Design review of the part built by this model. Coordinates are the model's own, in mm. Face numbers are marked on the shaded views. A direction names the side the tool comes from. Coordinates: 2 decimals unless noted, no trailing zeros. Write each loop counter-clockwise with the first axis right and the second up, starting at its lowest first coordinate (ties: lowest second). Pieces come first, ordered by that corner, then holes.
Autodesk Inventor part; units mm, degrees
ref_plane "YZ Plane" through (0, 0, 0) normal (1, 0, 0) x (0, 1, 0)
ref_plane "XZ Plane" through (0, 0, 0) normal (0, 1, 0) x (-1, 0, 0)
ref_plane "XY Plane" through (0, 0, 0) normal (0, 0, 1) x (1, 0, 0)
sketch "Sketch1" plane through (0, 0, 0) normal (0, 1, 0) x (-1, 0, 0)
  line L0 (20, -4.85) -> (-20, -4.85) construction
  line L1 (-20, -4.85) -> (-20, 4.85) construction
  line L2 (-20, 4.85) -> (20, 4.85) construction
  line L3 (20, 4.85) -> (20, -4.85) construction
  line L4 (0, -4.85) -> (0, 4.85) construction
  line L5 (20, 0) -> (-20, 0) construction
  circle A0 centre (13.5, 0) radius 2.25
  circle A1 centre (-13.5, 0) radius 2.25
  line L6 (67, -18) -> (25, -18) construction
  line L7 (25, -18) -> (25, 18) construction
  line L8 (25, 18) -> (67, 18) construction
  line L9 (67, 18) -> (67, -18) construction
  line L10 (46, -18) -> (46, 18) construction
  line L11 (67, 0) -> (25, 0) construction
  circle A2 centre (61.25, -13) radius 2.75
  circle A3 centre (30.75, -13) radius 2.75
  circle A4 centre (61.25, 13) radius 2.75
  circle A5 centre (30.75, 13) radius 2.75
  line L12 (-67, -18) -> (-25, -18) construction
  line L13 (-25, -18) -> (-25, 18) construction
  line L14 (-25, 18) -> (-67, 18) construction
  line L15 (-67, 18) -> (-67, -18) construction
  line L16 (-46, -18) -> (-46, 18) construction
  line L17 (-67, 0) -> (-25, 0) construction
  circle A6 centre (-61.25, -13) radius 2.75
  circle A7 centre (-30.75, -13) radius 2.75
  circle A8 centre (-61.25, 13) radius 2.75
  circle A9 centre (-30.75, 13) radius 2.75
  line L18 (82, -65) -> (-82, -65)
  line L19 (-82, -65) -> (-82, 65)
  line L20 (-82, 65) -> (82, 65)
  line L21 (82, 65) -> (82, -65)
  point P0 (0, 0)
  point P1 (0, 0)
  dimension "d0" = 40
  dimension "d1" = 9.7
  dimension "d2" = 4.5
  dimension "d3" = 27
  dimension "d4" = 42
  dimension "d6" = 36
  dimension "d7" = 5
  dimension "d8" = 5.5
  dimension "d9" = 30.5
  dimension "d10" = 26
  dimension "d12" = 15
  dimension "d16" = 130
extrude "Extrusion1" add sketch "Sketch1" along normal blind 10
sketch "Sketch5" plane through (-82, 0, -65) normal (-1, 0, 0) x (0, 0, 1)
  line L0 (0, 0) -> (130, 0)
  line L1 (130, 0) -> (130, 10)
  line L2 (0, 10) -> (130, 10)
  line L3 (0, 0) -> (0, 10)
  point P0 (65, 0)
extrude "Extrusion4" add sketch "Sketch5" along normal blind 10
sketch "Sketch6" plane through (0, 10, 0) normal (0, 1, 0) x (1, 0, 0)
  line L0 (-92, 65) -> (-92, -65)
  line L1 (82, -65) -> (-92, -65)
  line L2 (-92, 65) -> (-82, 65)
  line L3 (-82, 65) -> (-82, -65)
  line L4 (-82, -65) -> (-92, -65)
  line L5 (-92, -65) -> (-92, 65)
  point P0 (0, 0)
  dimension "d33" = 10
extrude "Extrusion5" add sketch "Sketch6" along normal blind 80
sketch "Sketch7" plane through (-82, 10, 65) normal (1, 0, 0) x (0, 0, -1)
  line L0 (35, 10) -> (95, 10)
  line L1 (95, 10) -> (95, 70)
  line L2 (95, 70) -> (35, 70)
  line L3 (35, 70) -> (35, 10)
  line L4 (130, 80) -> (0, 80) construction
  line L5 (65, 80) -> (65, 0) construction
  line L6 (62.75, 0) -> (67.25, 0) construction
  line L7 (0, -10) -> (0, 80) construction
  line L8 (130, -10) -> (130, 80) construction
  line L9 (130, 40) -> (0, 40) construction
  point P0 (65, -10)
  dimension "d36" = 60
  dimension "d37" = 60
  dimension "d38" = 40
extrude "Extrusion6" add sketch "Sketch7" along normal blind 10
sketch "Sketch8" plane through (0, 90, 0) normal (0, 1, 0) x (1, 0, 0)
  line L0 (-92, 65) -> (-92, -65)
  line L1 (-92, -65) -> (-82, -65)
  line L2 (-82, -65) -> (-82, 65)
  line L3 (-82, 65) -> (-92, 65)
  point P0 (0, 0)
extrude "Extrusion7" cut sketch "Sketch8" against normal up to surface (10 mm away)
sketch "Sketch9" plane through (-72, 10, 65) normal (1, 0, 0) x (0, 0, -1)
  line L0 (95, 10) -> (95, 70) construction
  line L1 (95, 70) -> (35, 70) construction
  line L2 (35, 70) -> (35, 10) construction
  line L3 (35, 10) -> (95, 10) construction
  line L4 (35, 10) -> (35, 70) construction
  line L5 (35, 40) -> (95, 40) construction
  line L6 (95, 10) -> (95, 70) construction
  line L7 (35, 10) -> (95, 10) construction
  line L8 (65, 10) -> (65, 70) construction
  line L9 (95, 70) -> (35, 70) construction
  line L10 (41.45, 63.55) -> (88.55, 63.55) construction
  line L11 (88.55, 63.55) -> (88.55, 16.45) construction
  line L12 (88.55, 16.45) -> (41.45, 16.45) construction
  line L13 (41.45, 16.45) -> (41.45, 63.55) construction
  circle A0 centre (41.45, 63.55) radius 2.75
  circle A1 centre (41.45, 16.45) radius 2.75
  circle A2 centre (88.55, 16.45) radius 2.75
  circle A3 centre (88.55, 63.55) radius 2.75
  circle A4 centre (65, 40) radius 19.05
  point P0 (65, -10)
  dimension "d43" = 47.1
  dimension "d44" = 47.1
  dimension "d45" = 5.5
  dimension "d46" = 5.5
  dimension "d47" = 5.5
  dimension "d48" = 5.5
  dimension "d51" = 38.1
extrude "Extrusion8" cut sketch "Sketch9" against normal through all
sketch "Sketch10" plane through (-92, 0, -65) normal (-1, 0, 0) x (0, 0, 1)
  circle A0 centre (65, 50) radius 19.05
  line L0 (65, 50) -> (0, 50) construction
  line L1 (0, 10) -> (0, 80)
  line L2 (65, 50) -> (130, 50) construction
  line L3 (130, 10) -> (130, 80)
  line L4 (5, 71.2) -> (33, 71.2) construction
  line L5 (33, 71.2) -> (33, 24.2) construction
  line L6 (33, 24.2) -> (5, 24.2) construction
  line L7 (5, 24.2) -> (5, 71.2) construction
  line L8 (5, 47.7) -> (33, 47.7) construction
  line L9 (65, 50) -> (65, 0) construction
  line L10 (19, 71.2) -> (19, 24.2) construction
  circle A1 centre (19, 65.7) radius 2.75
  circle A2 centre (19, 29.7) radius 2.75
  circle A3 centre (111, 65.7) radius 2.75
  circle A4 centre (111, 29.7) radius 2.75
  point P0 (180, 80)
  dimension "d52" = 28
  dimension "d53" = 47
  dimension "d54" = 2.3
  dimension "d55" = 46
  dimension "d56" = 5.5
  dimension "d57" = 36
extrude "Extrusion9" cut sketch "Sketch10" against normal through all contours A1 | A2 | A3 | A4
sketch "Sketch12" plane through (0, 10, 0) normal (0, 1, 0) x (1, 0, 0)
  line L0 (82, 65) -> (-82, 65)
  line L1 (-82, 65) -> (0, 65)
  line L2 (0, 65) -> (0, 55)
  line L3 (0, 55) -> (-82, 55)
  line L4 (-82, 55) -> (-82, 65)
  line L5 (82, -65) -> (82, 65) construction
  line L6 (82, 0) -> (-92, 0) construction
  line L7 (-92, 65) -> (-92, -65) construction
  line L8 (-82, -65) -> (0, -65)
  line L9 (0, -65) -> (0, -55)
  line L10 (0, -55) -> (-82, -55)
  line L11 (-82, -55) -> (-82, -65)
  point P0 (0, 0)
  dimension "d70" = 82
  dimension "d71" = 10
extrude "Extrusion11" add sketch "Sketch12" along normal up to surface (70 mm away)
chamfer "Chamfer3" distance 70 distance2 82 1 edges at (0, 80, -60) measured on face at (0, 33.3333, -58.3333)
chamfer "Chamfer4" distance 70 distance2 82 1 edges at (0, 80, 60) measured on face at (0, 33.3333, 61.6667)
sketch "Sketch13" plane through (-72, 10, 65) normal (1, 0, 0) x (0, 0, -1)
  line L0 (95, 10) -> (35, 10)
  line L1 (95, 10) -> (95, 70)
  line L2 (35, 10) -> (95, 10)
  line L3 (95, 10) -> (95, 70)
  line L4 (95, 70) -> (35, 70)
  line L5 (35, 70) -> (35, 10)
  point P0 (65, -10)
extrude "Extrusion12" add sketch "Sketch13" against normal blind 20
sketch "Sketch14" plane through (-72, 10, 65) normal (1, 0, 0) x (0, 0, -1)
  line L0 (95, 10) -> (95, 70)
  line L1 (95, 70) -> (35, 70)
  line L2 (35, 70) -> (35, 10)
  line L3 (35, 10) -> (95, 10)
  point P0 (65, -10)
extrude "Extrusion13" cut sketch "Sketch14" against normal blind 10
sketch "Sketch15" plane through (-92, 0, -65) normal (-1, 0, 0) x (0, 0, 1)
  circle A0 centre (19, 29.7) radius 2.75 construction
  circle A1 centre (19, 65.7) radius 2.75 construction
  line L0 (19, 29.7) -> (19, 65.7) construction
  circle A2 centre (111, 29.7) radius 2.75 construction
  circle A3 centre (111, 65.7) radius 2.75 construction
  line L1 (111, 29.7) -> (111, 65.7) construction
  line L2 (19, 47.7) -> (111, 47.7) construction
  line L3 (51.5, 74) -> (78.5, 74) construction
  line L4 (78.5, 74) -> (78.5, 26) construction
  line L5 (78.5, 26) -> (51.5, 26) construction
  line L6 (51.5, 26) -> (51.5, 74) construction
  line L7 (51.5, 50) -> (78.5, 50) construction
  line L8 (130, 80) -> (0, 80) construction
  line L9 (65, 80) -> (65, 0) construction
  line L10 (65, 74) -> (65, 26) construction
  circle A4 centre (65, 68.3) radius 2.75
  circle A5 centre (65, 31.7) radius 2.75
  dimension "d84" = 27
  dimension "d85" = 48
  dimension "d86" = 2.3
  dimension "d87" = 5.5
  dimension "d88" = 36.6
extrude "Extrusion14" cut sketch "Sketch15" against normal blind 10
properties part number "positioner_base"
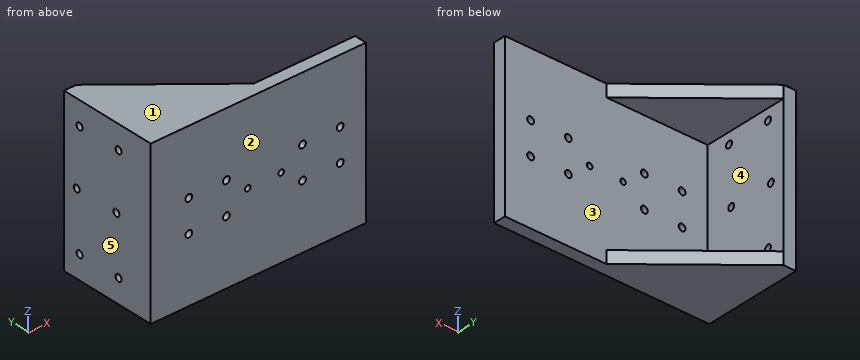
(1) Consider section A-A (z = 46). Give the boundary of the cut face in (x, y).
(2) Consider section D-D (y = 59). Give the boundary of the cut face in (x, z), plus the area to 3 significant figures.
(3) Consider section B-B (x = 13.5). Give the boundary of the cut face in (y, z), plus the area to 4 significant figures.
(4) Wall thickness on line 1 (Z direction, x = 61, y = 8); line 2 (Z direction, x = -80.5, y = 44); line 3 (Y direction, x = -1, z = -29.5): over which ranges is each line inside the solid? List them lowest first.
(5) Insertion check: pin 1 Ø6.5 at (x, z) = (61.25, -13) entering from +Y; pin 2 Ø2 at (y, z) = (40, -47.5) entering from +X. Each pin has a flat end and moves straight along its axis. Give the tip position at first contact, or say it passes through.
(6) For the marked faces 4 and 5, list the 3-axis set-ups (+Z, -Z, +X, -X, +Y, -Y) from which the entire face can be reached by the end or side of a thin tool; tool diameter is ignored.
(7) Consider section C-C (z = -13). Give the boundary of the cut face in (x, y).
(8) Mouldability with a two-part tool opening along Z and no side actions: class the marked faces 1, 2 and 3 as +Z half, -Z half, draft (parallel to the pull), parting line (faces both ways), or undercut.
Results:
1. outline: (-92, 0) - (82, 0) - (82, 10) - (-82, 10) - (-82, 26.95) - (-92, 26.95) - close; (-92, 32.45) - (-82, 32.45) - (-82, 62.95) - (-92, 62.95) - close; (-92, 68.45) - (-82, 68.45) - (-82, 80) - (-92, 80) - close
2. outline: (-92, -65) - (-57.4, -65) - (-57.4, -55) - (-82, -55) - (-82, 55) - (-57.4, 55) - (-57.4, 65) - (-92, 65) - close
2. area: 1,790 mm2
3. outline: (0, -65) - (10, -65) - (10, -2.25) - (0, -2.25) - close; (0, 2.25) - (10, 2.25) - (10, 65) - (0, 65) - close
3. area: 1,255 mm2
4. line 1: z = -65 to -15.74, -10.26 to 10.26, 15.74 to 65
4. line 2: z = -65 to -55, 55 to 65
4. line 3: y = 0 to 10
5. pin 1: stops at y = 10
5. pin 2: stops at x = -82
6. face 4: +X, +Y
6. face 5: +Z, -Z, -X, +Y, -Y
7. outline: (-92, 0) - (-64, 0) - (-64, 10) - (-82, 10) - (-82, 80) - (-92, 80) - close; (-58.5, 0) - (-33.5, 0) - (-33.5, 10) - (-58.5, 10) - close; (-28, 0) - (28, 0) - (28, 10) - (-28, 10) - close; (33.5, 0) - (58.5, 0) - (58.5, 10) - (33.5, 10) - close; (64, 0) - (82, 0) - (82, 10) - (64, 10) - close
8. face 1: +Z half
8. face 2: draft
8. face 3: undercut
